Geometry check sheet. Reference: the model listing, model coordinates, mm. A direction names the side the tool comes from. Round coordinates to 2 decimals unless told otherwise and drop trailing zeros. Order: outer loops, then holes, each group sorted by start corner. A loop starts at its lowest first (then second) coordinate and runs counter-clockwise, first axis right, second up. Notation, with made-up numbers: (65.5, 26) - (114.5, 26) arc R19 ccw to (114.5, 50) - close; hole circle Ø6 at (-39.75, 9.25). An arc over 180 degrees is marked (long way). Return JSON: item names as keys, results as strings. Group by question number.
Q1. Gauge pin test, flat ends, axial feed: pin 1 Ø19 at (x, z) = (12.5, 40.5) entering from +Y; pin 2 Ø2 at (x, z) = (-6, 51) entering from +Y; pin 3 Ø0.8 at (x, y) = (1.5, 0.5) entering from +Z. Record the tip position at first contact, or that the pin passes through.
Q2. Sectioned sample at D-D, the plane z = 5.5. Record the cut outline in (x, y).
Q3. Sectioned sample at A-A, the plane y = -18.5. Record the cut outline in (x, z).
Q4. Material ranges on line 1 along Y through (x, z) = (20.5, 52.5); line 2 along X through (y, z) = (28, 19), recorded low to high.
Q5. Draft check along Y on faces 4 (the flat face through (-20.018, -31.832, 9.367)), 5 (the flat face through (-44, 0, 43)), 6 (the flat face through (-54, 1.25, 34)), 7 (the flat face through (11.832, -0.018, 9.367)). Enter one of: pulls with the +Y half, pulls with the -Y half, needs draft (parallel to the pull), parting line crosses it, or undercut.
Q6. Sectioned sample at C-C, the plane x = -14. Record the cut outline in (y, z), then the cut area to 3 significant figures.
Q7. Sectioned sample at B-B, the plane z = 42. Record the cut outline in (x, y).
Q8. Tool access check on faces 1 (the flat face through (-40.64, -5.69, 30.98)), 2 (the flat face through (2, 0, 17)), 3 (the flat face through (-25.69, 20.64, 30.98)). Record the directions out of +Z, -Z, +X, -X, +Y, -Y that give a thin tool (end or side, any length) a straight path to the whole face; none if there is none.
```python
from build123d import *

# Parameters (mm, degrees)
F1_DEPTH  = 1.25
F3_COUNT  = 4
F6_DEPTH  = 45
F8_DEPTH  = 5
F9_COUNT  = 4
F11_DEPTH = 17


with BuildPart() as f1:
    # F0 (on Front) → F1 (new body, symmetric)
    with BuildSketch(Plane.XZ):
        with BuildLine():
            Line((0, 17), (0, 0))
            Line((0, 0), (24, 19))
            Line((24, 19), (24, 63))
            ThreePointArc((24, 63), (22.5355339059, 66.5355339059), (19, 68))
            Line((19, 68), (4, 68))
            Line((4, 68), (4, 17))
            Line((4, 17), (0, 17))
        make_face()
    extrude(amount=F1_DEPTH, both=True)


with BuildPart() as f3_1:
    # F3: instance of F1
    add(f1.part.rotate(Axis((-20, 0, 4.0539303016), (0, 0, 1)), 1 * 360 / F3_COUNT))


with BuildPart() as f3_2:
    # F3: instance of F1
    add(f1.part.rotate(Axis((-20, 0, 4.0539303016), (0, 0, 1)), 2 * 360 / F3_COUNT))


with BuildPart() as f3_3:
    # F3: instance of F1
    add(f1.part.rotate(Axis((-20, 0, 4.0539303016), (0, 0, 1)), 3 * 360 / F3_COUNT))


with BuildPart() as f6:
    # F5 (on face) → F6 (new body)
    with BuildSketch(Plane.XY.offset(68)):
        Polygon((-18.75, 26.1213203436), (-18.75, 24), (4, 1.25), (6.1213203436, 1.25), align=None)
    extrude(amount=-F6_DEPTH)

    # F7 (on face) → F8 (cut)
    with BuildSketch(Plane(origin=(3.6856601718, 3.6856601718, 0), x_dir=(-0.7071067812, 0.7071067812, 0), z_dir=(0.7071067812, 0.7071067812, 0))):
        with BuildLine():
            Line((31.7288148957, 23), (17.8969432153, 38.7299413567))
            ThreePointArc((17.8969432153, 38.7299413567), (14.1421356237, 40.4282115146), (10.3873280321, 38.7299413567))
            Line((10.3873280321, 38.7299413567), (-3.4445436483, 23))
            Line((-3.4445436483, 23), (31.7288148957, 23))
        make_face()
    extrude(amount=-F8_DEPTH, mode=Mode.SUBTRACT)


with BuildPart() as f1_1:
    add(f1.part)

    add(f3_1.part)  # F9 merges F3_1

    add(f3_2.part)  # F9 merges F3_2

    add(f3_3.part)  # F9 merges F3_3
    # F9: F6 ×4 about axis
    f9_axis = Axis((-20, 0, 68), (0, 0, 1))
    for i in range(1, F9_COUNT):
        add(f6.part.rotate(f9_axis, i * 360 / F9_COUNT))

    add(f6.part)  # F11 merges F6
    # F10 (on face) → F11 (join)
    with BuildSketch(Plane.XY.offset(17)):
        with BuildLine():
            Line((-18.75, 19.9608992783), (-18.75, 20))
            Line((-18.75, 20), (-19.9999998635, 20))
            ThreePointArc((-19.9999998635, 20), (-19.3746942332, 19.9902224274), (-18.75, 19.9608992783))
        make_face()
        with BuildLine():
            ThreePointArc((-21.25, 19.9608992783), (-20.6253056303, 19.9902224317), (-19.9999998635, 20))
            Line((-19.9999998635, 20), (-21.25, 20))
            Line((-21.25, 20), (-21.25, 19.9608992783))
        make_face()
        with BuildLine():
            Line((-0.0391007217, -1.25), (0, -1.25))
            Line((0, -1.25), (0, 9.88e-08))
            ThreePointArc((0, 9.88e-08), (-0.0097775689, -0.6253056492), (-0.0391007217, -1.25))
        make_face()
        with BuildLine():
            ThreePointArc((-0.0391007217, 1.25), (-0.009777572, 0.6253057479), (0, 9.88e-08))
            Line((0, 9.88e-08), (0, 1.25))
            Line((0, 1.25), (-0.0391007217, 1.25))
        make_face()
        with BuildLine():
            Line((-21.25, -19.9608992783), (-21.25, -20))
            Line((-21.25, -20), (-20.0000001365, -20))
            ThreePointArc((-20.0000001365, -20), (-20.6253057668, -19.9902224274), (-21.25, -19.9608992783))
        make_face()
        with BuildLine():
            ThreePointArc((-18.75, -19.9608992783), (-19.3746943697, -19.9902224317), (-20.0000001365, -20))
            Line((-20.0000001365, -20), (-18.75, -20))
            Line((-18.75, -20), (-18.75, -19.9608992783))
        make_face()
        with BuildLine():
            Line((-39.9608992783, 1.25), (-40, 1.25))
            Line((-40, 1.25), (-40, 0))
            ThreePointArc((-40, 0), (-39.9902224296, 0.6253056985), (-39.9608992783, 1.25))
        make_face()
        with BuildLine():
            ThreePointArc((-39.9608992783, -1.25), (-39.9902224296, -0.6253056985), (-40, 0))
            Line((-40, 0), (-40, -1.25))
            Line((-40, -1.25), (-39.9608992783, -1.25))
        make_face()
    extrude(amount=-F11_DEPTH)


solid = f1_1.part
```
Reply:
{
 "1": {"pin 1": "y = 4.37", "pin 2": "y = 14.37", "pin 3": "z = 17"},
 "2": {"outline": "(-46.95, -1.25) - (-39.96, -1.25) arc R20 cw to (-39.96, 1.25) - (-46.95, 1.25) - close; (-21.25, -26.95) - (-18.75, -26.95) - (-18.75, -19.96) arc R20 cw to (-21.25, -19.96) - close; (-21.25, 19.96) arc R20 cw to (-18.75, 19.96) - (-18.75, 26.95) - (-21.25, 26.95) - close; (-0.04, -1.25) - (6.95, -1.25) - (6.95, 1.25) - (-0.04, 1.25) arc R20 cw to start"},
 "3": {"outline": "(-28.87, 35.26) - (-26.75, 33.55) - (-26.75, 68) - (-28.87, 68) - close; (-13.25, 33.55) - (-11.13, 35.26) - (-11.13, 68) - (-13.25, 68) - close"},
 "4": {"line 1": "-1.25 to 1.25", "line 2": "-21.25 to -18.75"},
 "5": {"face 4": "pulls with the -Y half", "face 5": "undercut", "face 6": "pulls with the +Y half", "face 7": "needs draft"},
 "6": {"outline": "(-21.37, 30.64) - (-19.25, 32.35) - (-19.25, 68) - (-21.37, 68) - close; (19.25, 32.35) - (21.37, 30.64) - (21.37, 68) - (19.25, 68) - close", "area": "155 mm^2"},
 "7": {"outline": "(-64, -1.25) - (-46.12, -1.25) - (-21.25, -26.12) - (-21.25, -44) - (-18.75, -44) - (-18.75, -26.12) - (6.12, -1.25) - (24, -1.25) - (24, 1.25) - (6.12, 1.25) - (-18.75, 26.12) - (-18.75, 44) - (-21.25, 44) - (-21.25, 26.12) - (-46.12, 1.25) - (-64, 1.25) - close; hole (-44, -1.25) - (-21.25, -24) - (-18.75, -24) - (4, -1.25) - (4, 1.25) - (-18.75, 24) - (-21.25, 24) - (-44, 1.25) - close"},
 "8": {"face 1": "-Z, -Y", "face 2": "+Z, +Y, -Y", "face 3": "-Z, -X"}
}
